Design review of the part built by this model. Coordinates are the model's own, in mm. Face numbers are marked on the shaded views. A direction names the side the tool comes from. Coordinates: 2 decimals unless noted, no trailing zeros. Loops run counter-clockwise (first coordinate to the right, second up) from the corner with the lowest first, then second, coordinate; pieces in that order, holes last. Notation, with made-up numbers: (-29.5, -9.5) - (-1.5, -9.5) arc R13 cw to (-1.5, 2.5) - close; hole circle Ø4 at (57.5, 63). An arc over 180 degrees is marked (long way). One line per question, with ' | ' between items.
from build123d import *

# Parameters (mm, degrees)
F2_SIZE  = 0.5
F3_SIZE  = 0.5
F5_DEPTH = 1


with BuildPart() as f1:
    # F0 (on Front) → F1 (revolve)
    with BuildSketch(Plane.XZ):
        Polygon((0, 8), (0, 0), (2, 0), (2, 2), (3.9999996265, 2), (3.9999996265, 8), align=None)
    revolve(axis=Axis((0, 0, 4), (0, 0, -1)))

    # F2
    f2_edges = [f1.edges().sort_by_distance(p)[0] for p in [
        (-4, 0, 8),
    ]]
    chamfer(f2_edges, length=F2_SIZE)

    # F3
    f3_edges = [f1.edges().sort_by_distance(p)[0] for p in [
        (-4, 0, 2),
    ]]
    chamfer(f3_edges, length=F3_SIZE)

    # F4 (on face) → F5 (cut)
    with BuildSketch(Plane.XY.offset(8)):
        with BuildLine():
            Line((5, 0.5), (3.4641012378, 0.5))
            ThreePointArc((3.4641012378, 0.5), (3.4910134935, 0.2506435189), (3.4999996265, 0))
            ThreePointArc((3.4999996265, 0), (3.4910134935, -0.2506435189), (3.4641012378, -0.5))
            Line((3.4641012378, -0.5), (5, -0.5))
            Line((5, -0.5), (5, 0))
            Line((5, 0), (5, 0.5))
        make_face()
        with BuildLine():
            ThreePointArc((-3.4641012378, 0.5), (-3.4910134935, 0.2506435189), (-3.4999996265, 0))
            ThreePointArc((-3.4999996265, 0), (-3.4910134935, -0.2506435189), (-3.4641012378, -0.5))
            Line((-3.4641012378, -0.5), (3.4641012378, -0.5))
            ThreePointArc((3.4641012378, -0.5), (3.4910134935, -0.2506435189), (3.4999996265, 0))
            ThreePointArc((3.4999996265, 0), (3.4910134935, 0.2506435189), (3.4641012378, 0.5))
            Line((3.4641012378, 0.5), (-3.4641012378, 0.5))
        make_face()
        with BuildLine():
            ThreePointArc((-3.4641012378, -0.5), (-3.4910134935, -0.2506435189), (-3.4999996265, 0))
            Line((-3.4999996265, 0), (-5, 0))
            Line((-5, 0), (-5, -0.5))
            Line((-5, -0.5), (-3.4641012378, -0.5))
        make_face()
        with BuildLine():
            Line((-5, 0), (-3.4999996265, 0))
            ThreePointArc((-3.4999996265, 0), (-3.4910134935, 0.2506435189), (-3.4641012378, 0.5))
            Line((-3.4641012378, 0.5), (-5, 0.5))
            Line((-5, 0.5), (-5, 0))
        make_face()
    extrude(amount=-F5_DEPTH, mode=Mode.SUBTRACT)


solid = f1.part
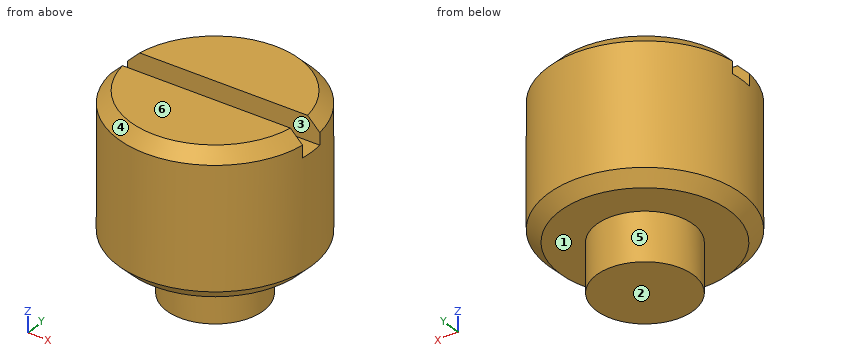
Q1. Take a section at A-A (y = 0). Give the boundary of the cut face in (x, z).
Returned:
outline: (-4, 2.5) - (-3.5, 2) - (-2, 2) - (-2, 0) - (2, 0) - (2, 2) - (3.5, 2) - (4, 2.5) - (4, 7) - (-4, 7) - close
Q2. For pin 1 (3 mm diameter, centred on y = 3, z = 2.5, fed in from -X); pin 2 (1.1 mm diameter, centred on x = 1, z = 7.5, fed in from +Y); pin 3 (1.5 mm diameter, centred on x = 1.5, z = 1, fed in from +Y), all flat-tipped, find the tip position at first contact; note any pin that passes through.
Returned:
pin 1: stops at x = -3.71 | pin 2: stops at y = 3.97 | pin 3: stops at y = 1.85
Q3. Take a section at C-C (x = 0). Give the boundary of the cut face in (y, z).
Returned:
outline: (-4, 2.5) - (-3.5, 2) - (-2, 2) - (-2, 0) - (2, 0) - (2, 2) - (3.5, 2) - (4, 2.5) - (4, 7.5) - (3.5, 8) - (0.5, 8) - (0.5, 7) - (-0.5, 7) - (-0.5, 8) - (-3.5, 8) - (-4, 7.5) - close
Q4. Tool access review of the marked faces 1 and 2: name each direction out of +Z, -Z, +X, -X, +Y, -Y from which nothing blocks a thin tool from reaching the whole face with its end or side.
Returned:
face 1: -Z | face 2: -Z, +X, -X, +Y, -Y
Q5. To check wall thickness, follow line 1 along Y through (x, z) = (-0.5, 6.5); line 2 along Z through (x, y) = (2, 1.5); line 3 along Y through (x, z) = (2, 3.5). State the ranges of each line that lie inside material, in increasing order.
Returned:
line 1: y = -3.97 to 3.97 | line 2: z = 2 to 8 | line 3: y = -3.46 to 3.46
Q6. Take a section at B-B (z = 7.25). Give the boundary of the cut face in (x, y), plus the area to 3 significant figures.
Returned:
outline: (-3.97, -0.5) arc R4 ccw to (3.97, -0.5) - close; (-3.97, 0.5) - (3.97, 0.5) arc R4 ccw to start | area: 42.3 mm²
Q7. Draft analysis for pull direction Y (two halves, no side actions). For the marked faces 3, 4, 5 and 6, state which applies: +Y half, -Y half, draft (parallel to the pull), parting line (faces both ways), or undercut.
Returned:
face 3: undercut | face 4: -Y half | face 5: parting line | face 6: draft
Q8. Take a section at D-D (z = 1). Give the boundary of the cut face in (x, y).
Returned:
outline: circle Ø4 at (0, 0)
